from build123d import *

# Parameters (mm, degrees)
SKETCH1_W           = 92
SKETCH1_H           = 31
BOSS_EXTRUDE2_DEPTH = 3
SKETCH1_3_W         = 100
SKETCH1_3_H         = 39
SKETCH1_3_W_2       = 92
SKETCH1_3_H_2       = 31
BOSS_EXTRUDE3_DEPTH = 73
FILLET1_R           = 2
FILLET2_R           = 2
SKETCH3_W           = 7.14
SKETCH3_H           = 31
BOSS_EXTRUDE4_DEPTH = 28
SKETCH4_W           = 7.14
SKETCH4_H           = 2.85103565
BOSS_EXTRUDE5_DEPTH = 4
SKETCH5_W           = 7.14
SKETCH5_H           = 5.56896435
CUT_EXTRUDE1_DEPTH  = 28
SKETCH4_3_R         = 0.5
CUT_EXTRUDE3_DEPTH  = 20
LPATTERN5_COUNT     = 2
LPATTERN5_PITCH     = 47.64
LPATTERN6_COUNT     = 2
LPATTERN6_PITCH     = 49
SKETCH10_W          = 2.85103565
SKETCH10_H          = 32
BOSS_EXTRUDE6_DEPTH = 41
CUT_EXTRUDE4_DEPTH  = 10


with BuildPart() as part:
    # Sketch1 → Boss-Extrude2 (new body)
    with BuildSketch(Plane(origin=(0, 0, 0), x_dir=(1, 0, 0), z_dir=(0, 1, 0))):
        Rectangle(SKETCH1_W, SKETCH1_H)
    extrude(amount=BOSS_EXTRUDE2_DEPTH)

    # Sketch1_3 → Boss-Extrude3 (add)
    with BuildSketch(Plane(origin=(0, 0, 0), x_dir=(1, 0, 0), z_dir=(0, 1, 0))):
        Rectangle(SKETCH1_3_W, SKETCH1_3_H)
        Rectangle(SKETCH1_3_W_2, SKETCH1_3_H_2, mode=Mode.SUBTRACT)
    extrude(amount=BOSS_EXTRUDE3_DEPTH)

    # Fillet1
    fillet1_edges = [part.edges().sort_by_distance(p)[0] for p in [
        (50, 36.5, 19.5),
    ]]
    fillet(fillet1_edges, radius=FILLET1_R)

    # Fillet2
    fillet2_edges = [part.edges().sort_by_distance(p)[0] for p in [
        (50, 36.5, -19.5),
    ]]
    fillet(fillet2_edges, radius=FILLET2_R)

    # Sketch3 → Boss-Extrude4 (add)
    with BuildSketch(Plane(origin=(0, 3, 0), x_dir=(1, 0, 0), z_dir=(0, 1, 0))):
        with Locations((42.43, 0)):
            Rectangle(SKETCH3_W, SKETCH3_H)
    boss_extrude4 = extrude(amount=BOSS_EXTRUDE4_DEPTH)

    # Sketch4 → Boss-Extrude5 (add)
    with BuildSketch(Plane(origin=(0, 31, 0), x_dir=(1, 0, 0), z_dir=(0, 1, 0))):
        with Locations((42.43, -8.505517825)):
            Rectangle(SKETCH4_W, SKETCH4_H)
    boss_extrude5 = extrude(amount=BOSS_EXTRUDE5_DEPTH)

    # Sketch5 → Cut-Extrude1 (cut)
    with BuildSketch(Plane(origin=(0, 31, 0), x_dir=(1, 0, 0), z_dir=(0, 1, 0))):
        with Locations((42.43, -12.715517825)):
            Rectangle(SKETCH5_W, SKETCH5_H)
    cut_extrude1 = extrude(amount=-CUT_EXTRUDE1_DEPTH, mode=Mode.SUBTRACT)

    # Sketch4_3 → Cut-Extrude3 (cut)
    with BuildSketch(Plane(origin=(0, 31, 0), x_dir=(1, 0, 0), z_dir=(0, 1, 0))):
        with Locations(Location((43.36, 8.92, 0), (0, 0, 270))):
            Circle(SKETCH4_3_R)
        with Locations(Location((43.36, -1.08, 0), (0, 0, 270))):
            Circle(SKETCH4_3_R)
    cut_extrude3 = extrude(amount=-CUT_EXTRUDE3_DEPTH, mode=Mode.SUBTRACT)

    # LPattern5: Boss-Extrude4, Boss-Extrude5, Cut-Extrude1 ×2
    with Locations(*[(-i * LPATTERN5_PITCH, 0, 0) for i in range(1, LPATTERN5_COUNT)]):
        add(boss_extrude4)
        add(boss_extrude5)
        add(cut_extrude1, mode=Mode.SUBTRACT)

    # LPattern6: Cut-Extrude3 ×2
    with Locations(*[(-i * LPATTERN6_PITCH, 0, 0) for i in range(1, LPATTERN6_COUNT)]):
        add(cut_extrude3, mode=Mode.SUBTRACT)

    # Sketch10 → Boss-Extrude6 (add)
    with BuildSketch(Plane.ZY.offset(-38.86)):
        with Locations((8.505517825, 19)):
            Rectangle(SKETCH10_W, SKETCH10_H)
    extrude(amount=BOSS_EXTRUDE6_DEPTH)

    # Sketch12 → Cut-Extrude4 (cut)
    with BuildSketch(Plane(origin=(-46, 0, 0), x_dir=(0, 0, -1), z_dir=(1, 0, 0))):
        with BuildLine():
            ThreePointArc((-6, 50), (0, 44), (6, 50))
            Line((6, 50), (-6, 50))
        make_face()
        with BuildLine():
            Line((-6, 50), (6, 50))
            ThreePointArc((6, 50), (0, 56), (-6, 50))
        make_face()
    extrude(amount=-CUT_EXTRUDE4_DEPTH, mode=Mode.SUBTRACT)


solid = part.part
Geometry check sheet. Reference: the model listing, model coordinates, mm. A direction names the side the tool comes from. Coordinates: 2 decimals unless noted, no trailing zeros. Order: outer loops, then holes, each group sorted by start corner. A loop starts at its lowest first (then second) coordinate and runs counter-clockwise, first axis right, second up. Notation, with made-up numbers: M 85.5,74 L 134.5,74 A7 cw 134.5,86 Z; hole C 70.5,43.5 d2. An arc over 180 degrees is marked long. Use CSV: the item, a comma, the result in double quotes.
Item 1: Thickness scan on line 1 along X through (y, z) = (23, 1); line 2 along X through (y, z) = (11.5, -14); line 3 along Z through (x, y) = (-5, 32). Record the ranges inside material, lowest first.
Returned:
line 1,"x = -50 to -46, -8.78 to -6.13, -5.15 to -1.64, 38.86 to 42.87, 43.85 to 50"
line 2,"x = -50 to -46, -8.78 to -1.64, 38.86 to 50"
line 3,"z = -19.5 to -15.5, 7.08 to 9.93, 15.5 to 19.5"
Item 2: Cross-section at B-B on y = 50. Record the cut outline in (x, z).
Returned:
outline,"M -50,-19.5 L 48,-19.5 A2 ccw 50,-17.5 L 50,17.5 A2 ccw 48,19.5 L -50,19.5 L -50,6 L -46,6 L -46,15.5 L 46,15.5 L 46,-15.5 L -46,-15.5 L -46,-6 L -50,-6 Z"
Item 3: Cross-section at D-D on y = 24.5. Record the cut outline in (x, z), then the cut area to 3 significant figures.
Returned:
outline,"M -50,-19.5 L 48,-19.5 A2 ccw 50,-17.5 L 50,17.5 A2 ccw 48,19.5 L -50,19.5 Z; hole M -46,-15.5 L -8.78,-15.5 L -8.78,9.93 L 46,9.93 L 46,15.5 L -46,15.5 Z; hole C -5.64,-8.92 d1; hole C -5.64,1.08 d1; hole M -1.64,-15.5 L 38.86,-15.5 L 38.86,7.08 L -1.64,7.08 Z; hole C 43.36,-8.92 d1; hole C 43.36,1.08 d1"
area,"1,520 mm2"
Item 4: Gauge pin test, flat ends, axial feed: pin 1 Ø6 at (x, z) = (-8.5, 2.5) entering from -Y; pin 2 Ø2 at (x, z) = (-6.5, -4) entering from +Y; pin 3 Ø0.9 at (x, z) = (28, 8) entering from +Y; pin 4 Ø11 at (y, z) = (50, 0) entering from -X. Record the tip position at first contact, or that the pin passes through.
Returned:
pin 1,"stops at y = 0"
pin 2,"stops at y = 31"
pin 3,"stops at y = 35"
pin 4,"stops at x = 46"
Item 5: Cross-section at C-C on z = -1. Record the cut outline in (x, y), then the cut area to 3 significant figures.
Returned:
outline,"M -50,0 L 50,0 L 50,73 L 46,73 L 46,31 L 38.86,31 L 38.86,3 L -1.64,3 L -1.64,31 L -8.78,31 L -8.78,3 L -46,3 L -46,44.08 L -50,44.08 Z; M -50,55.92 L -46,55.92 L -46,73 L -50,73 Z"
area,"1,210 mm2"
Item 6: Tool access check on faces 1 (the cylindrical face through (-47.972, 44.143, 1.301)), 2 (the flat face through (-1, 0, 0)), 3 (the flat face through (-46, 38, 0)). Record the directions out of +Z, -Z, +X, -X, +Y, -Y that give a thin tool (end or side, any length) a straight path to the whole face; none if there is none.
Returned:
face 1,"-X"
face 2,"+Z, -Z, +X, -X, -Y"
face 3,"+Y"
Item 7: Cross-section at A-A on x = 18. Record the cut outline in (y, z).
Returned:
outline,"M 0,-19.5 L 73,-19.5 L 73,-15.5 L 3,-15.5 L 3,7.08 L 35,7.08 L 35,9.93 L 3,9.93 L 3,15.5 L 73,15.5 L 73,19.5 L 0,19.5 Z"
Item 8: Mould release check, pull along Z, two halves, no side actions. Record for faces 4 (the flat face through (-2, 36, 19.5)), 5 (the flat face through (19, 19, 7.08)), 6 (the flat face through (50, 36, 0)): pulls with the +Z half, pulls with the -Z half, needs draft (parallel to the pull), parting line crosses it, or undercut.
Returned:
face 4,"pulls with the +Z half"
face 5,"undercut"
face 6,"needs draft"
